```python
from build123d import *

# Parameters (mm, degrees)
BOSS_EXTRUDE1_DEPTH             = 50
CHAMFER1_SIZE                   = 7
SKETCH2_R                       = 3.5
CUT_EXTRUDE1_DEPTH              = 62.524385409
SKETCH3_R                       = 1.75
CUT_EXTRUDE2_DEPTH              = 62.524385409
SKETCH5_R                       = 12.5
CUT_EXTRUDE4_DEPTH              = 3
BOSS_EXTRUDE2_DEPTH             = 7
CUT_EXTRUDE3_DEPTH              = 77.547867994
CUT_EXTRUDE3_DEPTH_BACK         = 77.547867994
SKETCH4_W                       = 51
SKETCH4_H                       = 47
SKETCH7_R                       = 1.25
SKETCH7_R_2                     = 5
CUT_EXTRUDE5_DEPTH              = 103.505990745
SKETCH8_R                       = 14.5
CUT_EXTRUDE6_DEPTH              = 3
SKETCH9_R                       = 3
CUT_EXTRUDE7_DEPTH              = 2
SKETCH11_R                      = 2
CUT_EXTRUDE8_DEPTH              = 10
BOSS_EXTRUDE3_START             = -32.5
BOSS_EXTRUDE3_DEPTH             = 65
SKETCH12_R                      = 2.6
CUT_EXTRUDE9_DEPTH              = 105.684053225
CUT_EXTRUDE10_DEPTH             = 3
BOSS_EXTRUDE4_DEPTH             = 3
SKETCH16_R                      = 1.75
CUT_EXTRUDE12_DEPTH             = 8
CHAMFER2_SIZE                   = 10
CUT_EXTRUDE14_DEPTH             = 10
CUT_EXTRUDE15_DEPTH             = 89.260982281
CUT_EXTRUDE15_DEPTH_BACK        = 89.260982281
CUT_EXTRUDE16_REACH             = 90.261
SKETCH19_R                      = 11
CUT_EXTRUDE16_DIRECTION_2_REACH = 90.261


# Read off the part's stored shape, not the designer's step: Mirror1
with BuildPart() as part:
    # Sketch1 → Boss-Extrude1 (new body)
    with BuildSketch(Plane.XY):
        Polygon((-27.5, 0), (-27.5, 20), (0, 20), (0, 23), (-32.5, 23), (-32.5, 0), align=None)
    extrude(amount=BOSS_EXTRUDE1_DEPTH)

    # Chamfer1
    # the kernel refuses this chamfer: 7 mm, written as the material it takes off along each edge
    with BuildSketch(Plane(origin=(-32.5, 0, -18.001780916), x_dir=(-0.02749587661058612, 0.9996219169112968, 0), z_dir=(0, 0, 1))) as chamfer1_piece_1:
        Polygon((CHAMFER1_SIZE * 0.999621916911, -CHAMFER1_SIZE * 0.0274958766106), (-CHAMFER1_SIZE * 0.0274958766106, -CHAMFER1_SIZE * 0.999621916911), (0, 0), align=None)
    extrude(amount=86.003561832, mode=Mode.SUBTRACT)

    # Sketch2 → Cut-Extrude1 (cut, through all)
    with BuildSketch(Plane(origin=(-27.5, 0, 0), x_dir=(0, 0, -1), z_dir=(1, 0, 0))):
        with Locations((-35, 12)):
            Circle(SKETCH2_R)
    extrude(amount=-CUT_EXTRUDE1_DEPTH, mode=Mode.SUBTRACT)

    # Sketch3 → Cut-Extrude2 (cut, through all)
    with BuildSketch(Plane(origin=(-27.5, 0, 0), x_dir=(0, 0, -1), z_dir=(1, 0, 0))):
        with Locations((-10, 16)):
            Circle(SKETCH3_R)
        with Locations((-16, 16)):
            Circle(SKETCH3_R)
    extrude(amount=-CUT_EXTRUDE2_DEPTH, mode=Mode.SUBTRACT)

    # Sketch5 → Cut-Extrude4 (cut)
    with BuildSketch(Plane.ZY.offset(32.5)):
        with Locations((35, 12)):
            Circle(SKETCH5_R)
    extrude(amount=-CUT_EXTRUDE4_DEPTH, mode=Mode.SUBTRACT)

    # Sketch6 → Boss-Extrude2 (add)
    with BuildSketch(Plane.ZY.offset(32.5)):
        with BuildLine():
            Line((38.91656851, 42.559195759), (20, 23))
            Line((20, 23), (41.190648452, 23))
            ThreePointArc((41.190648452, 23), (45.305332833, 20.647646722), (50, 19.996268429))
            Line((50, 19.996268429), (50, 7))
            Line((50, 7), (61.474012963, 24.541456905))
            ThreePointArc((61.474012963, 24.541456905), (58.38884507, 43.808308659), (38.91656851, 42.559195759))
        make_face()
    extrude(amount=-BOSS_EXTRUDE2_DEPTH)

    # Mirror1: part across plane


with BuildPart() as part_1:
    add(part.part)
    add(part.part.mirror(Plane(origin=(0, 0, 0), x_dir=(0, 0, 1), z_dir=(1, 0, 0))))

    # Sketch4 → Cut-Extrude3 (cut, two sides: drawn at the far end of the back side and taken through both)
    with BuildSketch(Plane.XZ.offset(-20).offset(-CUT_EXTRUDE3_DEPTH_BACK)):
        with Locations((0, 26.5)):
            Rectangle(SKETCH4_W, SKETCH4_H)
    extrude(amount=CUT_EXTRUDE3_DEPTH + CUT_EXTRUDE3_DEPTH_BACK, mode=Mode.SUBTRACT)

    # Sketch7 → Cut-Extrude5 (cut, through all)
    with BuildSketch(Plane.ZY.offset(32.5)):
        with Locations(Location((41.557466488, 37.927777253, 0), (0, 0, 270))):
            Circle(SKETCH7_R)
        with Locations(Location((57.12135533, 27.029824962, 0), (0, 0, 270))):
            Circle(SKETCH7_R)
        with Locations(Location((47.6186816, 30.021344974, 0), (0, 0, 270))):
            Circle(SKETCH7_R_2)
    extrude(amount=-CUT_EXTRUDE5_DEPTH, mode=Mode.SUBTRACT)

    # Sketch8 → Cut-Extrude6 (cut)
    with BuildSketch(Plane.ZY.offset(32.5)):
        with Locations((47.6186816, 30.021344974)):
            Circle(SKETCH8_R)
    cut_extrude6 = extrude(amount=-CUT_EXTRUDE6_DEPTH, mode=Mode.SUBTRACT)

    # Sketch9 → Cut-Extrude7 (cut)
    with BuildSketch(Plane.ZY.offset(29.5)):
        with Locations(Location((41.557466488, 37.927777253, 0), (0, 0, 270))):
            Circle(SKETCH9_R)
        with Locations(Location((57.12135533, 27.029824962, 0), (0, 0, 270))):
            Circle(SKETCH9_R)
    cut_extrude7 = extrude(amount=-CUT_EXTRUDE7_DEPTH, mode=Mode.SUBTRACT)

    # Sketch11 → Cut-Extrude8 (cut)
    with BuildSketch(Plane(origin=(0, 0, 0), x_dir=(-1, 0, 0), z_dir=(0, 0, -1))):
        with Locations((-30, 15.523029521)):
            Circle(SKETCH11_R)
    cut_extrude8 = extrude(amount=-CUT_EXTRUDE8_DEPTH, mode=Mode.SUBTRACT)

    # Mirror2: Cut-Extrude6, Cut-Extrude7, Cut-Extrude8 across plane
    add(cut_extrude6.mirror(Plane(origin=(0, 0, 0), x_dir=(0, 0, 1), z_dir=(1, 0, 0))), mode=Mode.SUBTRACT)
    add(cut_extrude7.mirror(Plane(origin=(0, 0, 0), x_dir=(0, 0, 1), z_dir=(1, 0, 0))), mode=Mode.SUBTRACT)
    add(cut_extrude8.mirror(Plane(origin=(0, 0, 0), x_dir=(0, 0, 1), z_dir=(1, 0, 0))), mode=Mode.SUBTRACT)

    # Sketch10 → Boss-Extrude3 (add)
    with BuildSketch(Plane(origin=(0, 0, 0), x_dir=(0, 0, -1), z_dir=(1, 0, 0)).offset(BOSS_EXTRUDE3_START)):
        with BuildLine():
            Line((-38.91656851, 42.559195759), (-33.44256114, 36.899227268))
            ThreePointArc((-33.44256114, 36.899227268), (-53.026270805, 48.561620018), (-65.574367209, 29.533263138))
            Line((-65.574367209, 29.533263138), (-61.474012963, 24.541456905))
            ThreePointArc((-61.474012963, 24.541456905), (-58.38884507, 43.808308659), (-38.91656851, 42.559195759))
        make_face()
    extrude(amount=BOSS_EXTRUDE3_DEPTH)

    # Sketch12 → Cut-Extrude9 (cut, through all)
    with BuildSketch(Plane(origin=(32.5, 0, 0), x_dir=(0, 0, -1), z_dir=(1, 0, 0))):
        with Locations(Location((-10, 8, 0), (0, 0, 180))):
            Circle(SKETCH12_R)
    extrude(amount=-CUT_EXTRUDE9_DEPTH, mode=Mode.SUBTRACT)

    # Sketch13 → Cut-Extrude10 (cut)
    with BuildSketch(Plane(origin=(32.5, 0, 0), x_dir=(0, 0, -1), z_dir=(1, 0, 0))):
        with BuildLine():
            ThreePointArc((-13, 18.645751311), (-20, 16), (-13, 13.354248689))
            ThreePointArc((-13, 13.354248689), (-6, 16), (-13, 18.645751311))
        make_face()
    cut_extrude10 = extrude(amount=-CUT_EXTRUDE10_DEPTH, mode=Mode.SUBTRACT)

    # Mirror3: Cut-Extrude10 across plane
    add(cut_extrude10.mirror(Plane(origin=(0, 0, 0), x_dir=(0, 0, 1), z_dir=(1, 0, 0))), mode=Mode.SUBTRACT)

    # Sketch15 → Boss-Extrude4 (add)
    with BuildSketch(Plane(origin=(0, 0, 0), x_dir=(-1, 0, 0), z_dir=(0, 0, -1))):
        with BuildLine():
            Line((-14, 25), (-14, 23))
            Line((-14, 23), (-6, 23))
            Line((-6, 23), (-6, 25))
            ThreePointArc((-6, 25), (-10, 29), (-14, 25))
        make_face()
        with BuildLine():
            Line((6, 23), (6, 25))
            ThreePointArc((6, 25), (10, 29), (14, 25))
            Line((14, 25), (14, 23))
            Line((14, 23), (6, 23))
        make_face()
    extrude(amount=-BOSS_EXTRUDE4_DEPTH)

    # Sketch16 → Cut-Extrude12 (cut)
    with BuildSketch(Plane(origin=(0, 0, 0), x_dir=(-1, 0, 0), z_dir=(0, 0, -1))):
        with Locations((-10, 25)):
            Circle(SKETCH16_R)
        with Locations((10, 25)):
            Circle(SKETCH16_R)
    extrude(amount=-CUT_EXTRUDE12_DEPTH, mode=Mode.SUBTRACT)

    # Chamfer2
    chamfer2_edges = [part_1.edges().sort_by_distance(p)[0] for p in [
        (25.5, 21.5, 3),
        (-25.5, 21.5, 3),
    ]]
    chamfer(chamfer2_edges, length=CHAMFER2_SIZE)

    # Sketch17 → Cut-Extrude14 (cut)
    with BuildSketch(Plane(origin=(0, 0, 0), x_dir=(-1, 0, 0), z_dir=(0, 0, -1))):
        Polygon((-32.5, 18), (-32.5, 23), (-27.5, 23), align=None)
        Polygon((32.5, 23), (27.5, 23), (32.5, 18), align=None)
    extrude(amount=-CUT_EXTRUDE14_DEPTH, mode=Mode.SUBTRACT)

    # Sketch18 → Cut-Extrude15 (cut, two sides: drawn at the far end of the back side and taken through both)
    with BuildSketch(Plane(origin=(0, 0, 0), x_dir=(0, 0, -1), z_dir=(1, 0, 0)).offset(-CUT_EXTRUDE15_DEPTH_BACK)):
        with BuildLine():
            Line((-30.530550933, 2), (-50, 2))
            Line((-50, 2), (-58.261274719, 19.629826629))
            ThreePointArc((-58.261274719, 19.629826629), (-46.960735265, 6.780592155), (-30.530550933, 2))
        make_face()
    extrude(amount=CUT_EXTRUDE15_DEPTH + CUT_EXTRUDE15_DEPTH_BACK, mode=Mode.SUBTRACT)

    # Cut-Extrude16: up to this face of the body (flat: up to its plane)
    cut_extrude16_end = Plane(part_1.part.faces().sort_by_distance((-27.5, 11.293188811, 24.090581316))[0])
    # Sketch19 → Cut-Extrude16 (cut, up to the picked face)
    with BuildSketch(Plane(origin=(0, 0, 0), x_dir=(0, 0, -1), z_dir=(1, 0, 0)), mode=Mode.PRIVATE) as cut_extrude16_sk1:
        with Locations((-35, 12)):
            Circle(SKETCH19_R)
    cut_extrude16_tool1 = split(extrude(cut_extrude16_sk1.sketch, amount=-CUT_EXTRUDE16_REACH, mode=Mode.PRIVATE), bisect_by=cut_extrude16_end, keep=Keep.BOTH, mode=Mode.PRIVATE)
    add(cut_extrude16_tool1.solids().sort_by(Axis((0, 12, 35), (-1, 0, 0)))[0], mode=Mode.SUBTRACT)

    # Cut-Extrude16 direction 2: up to this face of the body (flat: up to its plane)
    cut_extrude16_direction_2_end = Plane(part_1.part.faces().sort_by_distance((27.5, 11.293188811, 24.090581316))[0])
    # Sketch19 → Cut-Extrude16 direction 2 (cut, up to the picked face)
    with BuildSketch(Plane(origin=(0, 0, 0), x_dir=(0, 0, -1), z_dir=(1, 0, 0)), mode=Mode.PRIVATE) as cut_extrude16_direction_2_sk1:
        with Locations((-35, 12)):
            Circle(SKETCH19_R)
    cut_extrude16_direction_2_tool1 = split(extrude(cut_extrude16_direction_2_sk1.sketch, amount=CUT_EXTRUDE16_DIRECTION_2_REACH, mode=Mode.PRIVATE), bisect_by=cut_extrude16_direction_2_end, keep=Keep.BOTH, mode=Mode.PRIVATE)
    add(cut_extrude16_direction_2_tool1.solids().sort_by(Axis((0, 12, 35), (1, 0, 0)))[0], mode=Mode.SUBTRACT)


solid = part_1.part
```
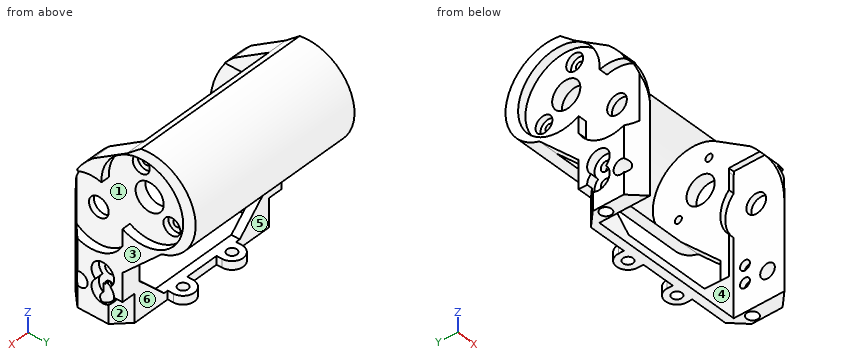
Source: CAD feature listing. Evaluate the final solid. Frame: model axes, mm. Face numbers are marked on the shaded views. A direction names the side the tool comes from. Coordinates: 2 decimals unless noted, no trailing zeros. Loops run counter-clockwise (first coordinate to the right, second up) from the corner with the lowest first, then second, coordinate; pieces in that order, holes last. Notation, with made-up numbers: (15, -17) -> (38, -17) arc R27 ccw to (38, 18) -> close; hole circle Ø1 at (15, 12.5). An arc over 180 degrees is marked (long way). One line per item, written item: value. Start each with the question number.
Q1. Section query C-C, the plane y = 33.5. Return the cut outline in (x, z).
Q2. Section query B-B, the plane x = -10. Return the cut outline in (y, z), and give its area (3 significant figures).
Q3. Section query A-A, the plane x = 5. Return the cut outline in (y, z).
Q4. Line query: line 1 along X through (y, z) = (23, 44); line 2 along X through (y, z) = (16.5, 54.5); line 3 along Y through (x, z) = (-30.6, 16). Output: solid intervals per line, ascending.
Q5. Contact query for flat-ended pins moving along their axis: P1, Ø4, axis at x = -18, z = 53.5, coming from the +Y side; P2, Ø1.8, axis at y = 36.5, z = 42, coming from the +X side; P3, Ø3, axis at x = 23, z = 29, coming from the +Y side; P4, Ø4, axis at y = 20, z = 37.5, coming from the -X side. Output: stop coordinate, or through.
Q6. Section query D-D, the plane z = 19. Return the cut outline in (x, y).
Q7. Mould query, pull axis Y, two halves, no side actions, for the marked faces 1, 2 and 3. Classes: pulls with the +Y half, pulls with the -Y half, needs draft (parallel to the pull), parting line crosses it, or undercut.
Q8. Set-up query: the marked faces 4, 5 and 6. Return all of +Z, -Z, +X, -X, +Y, -Y with unobstructed straight access to the full face (end or side cutting, diameter ignored); none if empty.
Results:
1. outline: (-32.5, 30.16) -> (-25.5, 30.16) -> (-25.5, 44.03) -> (-29.5, 44.03) -> (-29.5, 33.54) -> (-32.5, 33.54) -> close; (-32.5, 61.7) -> (-29.5, 61.7) -> (-29.5, 51.21) -> (-25.5, 51.21) -> (-25.5, 63.8) -> (25.5, 63.8) -> (25.5, 51.21) -> (29.5, 51.21) -> (29.5, 61.7) -> (32.5, 61.7) -> (32.5, 65.81) -> (-32.5, 65.81) -> close; (25.5, 30.16) -> (32.5, 30.16) -> (32.5, 33.54) -> (29.5, 33.54) -> (29.5, 44.03) -> (25.5, 44.03) -> close
2. outline: (20, 0) -> (23.25, 0) -> (23.25, 3) -> (20, 3) -> close; (24.54, 61.47) arc R14.5 cw to (42.56, 38.92) -> (36.9, 33.44) arc R16.5 ccw to (29.53, 65.57) -> close; (26.75, 0) -> (29, 0) -> (29, 3) -> (26.75, 3) -> close
2. area: 111 mm^2
3. outline: (20, 0) -> (23, 0) -> (23, 3) -> (20, 3) -> close; (24.54, 61.47) arc R14.5 cw to (42.56, 38.92) -> (36.9, 33.44) arc R16.5 ccw to (29.53, 65.57) -> close
4. line 1: -29.5 to -25.5, 25.5 to 29.5
4. line 2: -32.5 to -25.5, 25.5 to 32.5
4. line 3: 5.1 to 12, 20 to 23
5. P1: y = 48.84
5. P2: x = 27.5
5. P3: through
5. P4: x = -29.5
6. outline: (-32.5, 7) -> (-27.5, 2) -> (-27.5, 20) -> (-25.5, 20) -> (-25.5, 23) -> (-32.5, 23) -> (-32.5, 18.65) -> (-29.5, 18.65) -> (-29.5, 13.35) -> (-32.5, 13.35) -> close; (25.5, 20) -> (27.5, 20) -> (27.5, 2) -> (32.5, 7) -> (32.5, 13.35) -> (29.5, 13.35) -> (29.5, 18.65) -> (32.5, 18.65) -> (32.5, 23) -> (25.5, 23) -> close
7. face 1: undercut
7. face 2: pulls with the +Y half
7. face 3: needs draft
8. face 4: -Z, -Y
8. face 5: -Z, -X, +Y
8. face 6: -Z, +X, +Y
